Design review of the part built by this model. Coordinates are the model's own, in mm. A direction names the side the tool comes from. Coordinates: 2 decimals unless noted, no trailing zeros. Loops run counter-clockwise (first coordinate to the right, second up) from the corner with the lowest first, then second, coordinate; pieces in that order, holes last. Notation, with made-up numbers: (-38.75, -7.5) -> (16.25, -7.5) arc R21 cw to (16.25, -0.5) -> close; hole circle Ø3 at (-20.5, 17.25). An arc over 180 degrees is marked (long way). Use CSV: the item, a comma, the result in double quotes.
```python
from build123d import *

# Parameters (mm, degrees)
SKETCH1_R           = 2
SKETCH1_R_2         = 4
SKETCH1_R_3         = 1.25
SKETCH1_R_4         = 0.801632387
SKETCH1_R_5         = 1
BOSS_EXTRUDE1_DEPTH = 5
FILLET1_R           = 10
FILLET2_R           = 2
FILLET3_R           = 2


with BuildPart() as part:
    # Sketch1 → Boss-Extrude1 (new body)
    with BuildSketch(Plane(origin=(0, 0, 0), x_dir=(1, 0, 0), z_dir=(0, 1, 0))):
        with BuildLine():
            Line((10.245447832, 19.748535419), (14.245447832, 19.748535419))
            Line((14.245447832, 19.748535419), (14.245447832, 19.765232538))
            ThreePointArc((14.245447832, 19.765232538), (17.995447832, 16.015232538), (14.245447832, 12.265232538))
            Line((14.245447832, 12.265232538), (14.245447832, 12.251464581))
            Line((14.245447832, 12.251464581), (10.245447832, 12.251464581))
            ThreePointArc((10.245447832, 12.251464581), (8.910242614, 9.915125816), (7.000398069, 8.019408112))
            Line((7.000398069, 8.019408112), (7.000398069, 3.019408112))
            ThreePointArc((7.000398069, 3.019408112), (8.876398613, 0.90896847), (11.319846515, -0.506268567))
            ThreePointArc((11.319846515, -0.506268567), (15.105800834, -10.846250302), (10.471403603, -20.834795477))
            ThreePointArc((10.471403603, -20.834795477), (10.121274527, -21.168091922), (9.758861069, -21.487987805))
            ThreePointArc((9.758861069, -21.487987805), (7.187603365, -23.373618777), (4.217131367, -24.532612502))
            ThreePointArc((4.217131367, -24.532612502), (1.88896648, -24.924600666), (-0.415858892, -24.412949939))
            Line((-0.415858892, -24.412949939), (-7.21726234, -17.990260503))
            ThreePointArc((-7.21726234, -17.990260503), (-8.645604673, -16.078135797), (-9.343313072, -13.79568411))
            ThreePointArc((-9.343313072, -13.79568411), (-8.067302671, -0.037990819), (-8.771466645, 13.760794646))
            ThreePointArc((-8.771466645, 13.760794646), (-2.028677736, 25.538358263), (10.245447832, 19.748535419))
        make_face()
        Circle(SKETCH1_R, mode=Mode.SUBTRACT)
        with Locations((-0.296635989, -14.897704258)):
            Circle(SKETCH1_R_2, mode=Mode.SUBTRACT)
        with Locations((0.974607405, 16)):
            Circle(SKETCH1_R_3, mode=Mode.SUBTRACT)
        with Locations((10.245447832, 16.015232538)):
            Circle(SKETCH1_R_4, mode=Mode.SUBTRACT)
        with Locations((12.706975529, -10.846250302)):
            Circle(SKETCH1_R_5, mode=Mode.SUBTRACT)
    extrude(amount=BOSS_EXTRUDE1_DEPTH)

    # Fillet1
    fillet1_edges = [part.edges().sort_by_distance(p)[0] for p in [
        (11.319846515, 2.5, 0.506268567),
    ]]
    fillet(fillet1_edges, radius=FILLET1_R)

    # Fillet2
    fillet2_edges = [part.edges().sort_by_distance(p)[0] for p in [
        (7.000398069, 2.5, -3.019408112),
    ]]
    fillet(fillet2_edges, radius=FILLET2_R)

    # Fillet3
    fillet3_edges = [part.edges().sort_by_distance(p)[0] for p in [
        (-0.415858892, 2.5, 24.412949939),
    ]]
    fillet(fillet3_edges, radius=FILLET3_R)


solid = part.part
```
Item 1: Add section B-B (x = 8.5). Give the boundary of the cut face in (y, z).
Checked values:
outline,"(0, -22.59) -> (5, -22.59) -> (5, -9.41) -> (0, -9.41) -> close; (0, -1.23) -> (5, -1.23) -> (5, 22.54) -> (0, 22.54) -> close"
Item 2: To check wall thickness, follow line 1 along Z through (x, y) = (13.5, 1.45); line 2 along X through (y, z) = (2.85, -16); line 3 along Z through (x, y) = (0, 1.8). State the ranges of each line that lie inside material, in increasing order.
Checked values:
line 1,"-19.75 to -12.25, 3.62 to 10.24, 11.46 to 16.88"
line 2,"-9.03 to -0.28, 2.22 to 9.44, 11.05 to 18"
line 3,"-25.95 to -16.78, -15.22 to -2, 2 to 10.91, 18.89 to 24.58"
Item 3: Add section D-D (x = 13). State how many separate pieces and enclosed holes the cut face has, then the cut area to 3 significant figures.
Checked values:
separate pieces,"3"
enclosed holes,"0"
area,"103 mm^2"
Item 4: Add section A-A (z = 17). Give the boundary of the cut face in (x, y).
Checked values:
outline,"(-8.08, 0) -> (-3.7, 0) -> (-3.7, 5) -> (-8.08, 5) -> close; (3.11, 0) -> (13.43, 0) -> (13.43, 5) -> (3.11, 5) -> close"
Item 5: Machinability: for faces 4 (the face through (7, 2, -6)), 5 (the face through (7.23, 2.46, 23.35)), which of the approach directions +Z, -Z, +X, -X, +Y, -Y give a long, thin tool a straight path to every point of the face, cutting with its end or side? Answer none if there is none.
Checked values:
face 4,"+X, +Y, -Y"
face 5,"+Z, +X, +Y, -Y"
Item 6: Draft analysis for pull direction X (two halves, no side actions). For faces 1 (the face through (5, 5, -1)), 2 (the face through (8.9, 2.5, -9.9)), 3 (the face through (1.65, 2.46, -17.05)), state which applies: pulls with the +X half, pulls with the -X half, needs draft (parallel to the pull), parting line crosses it, or undercut.
Checked values:
face 1,"needs draft"
face 2,"pulls with the +X half"
face 3,"undercut"
Item 7: Add section C-C (z = 5.5). Give the boundary of the cut face in (x, y).
Checked values:
outline,"(-8.34, 0) -> (14.31, 0) -> (14.31, 5) -> (-8.34, 5) -> close"
Item 8: Clearance check with flat-ended pins moving along their axes: pin 1 (1 mm diameter, centred on y = 2.5, z = 8, fed in from -X); pin 2 (1.5 mm diameter, centred on y = 2.5, z = -12.5, fed in from +X); pin 3 (3 mm diameter, centred on x = 11.5, y = 1.5, fed in from +Z). State where each tip first meets the part, or that it passes through.
Checked values:
pin 1,"x = -8.62"
pin 2,"x = 16.78"
pin 3,"z = 21.28"
